Read the model definition and answer for the solid it produces. Units are mm, in the model's axes. A direction names the side the tool comes from. Give positions to 0.01 mm unless a question says otherwise; leave off trailing zeros. Order: outer loops, then holes, each group sorted by start corner. A loop starts at its lowest first (then second) coordinate and runs counter-clockwise, first axis right, second up. Notation, with made-up numbers: (57.25, 76.5) - (86.25, 76.5) arc R23 cw to (86.25, 87.5) - close; hole circle Ø4 at (6.5, 35.25). An arc over 180 degrees is marked (long way). Return JSON: item names as keys, results as strings.
```python
from build123d import *

# Parameters (mm, degrees)
SKETCH_1_W          = 45
SKETCH_1_H          = 80
EXTRUDE_1_DEPTH     = 6
CUT_EXTRUDE_2_DEPTH = 84.320165626
FILLET_10_R         = 2
M3X0_52_D           = 2.5
M3X0_52_DEPTH       = 8.5
M3X0_52_TIP         = 0.751075774
M3X0_51_D           = 2.5
M3X0_51_DEPTH       = 8.5
M3X0_51_TIP         = 0.751075774


with BuildPart() as part:
    # Эскиз1 → Бобышка-Вытянуть1 (new body)
    with BuildSketch(Plane(origin=(0, 0, 0), x_dir=(1, 0, 0), z_dir=(0, 1, 0))):
        with Locations((0, -40)):
            Rectangle(SKETCH_1_W, SKETCH_1_H)
    extrude(amount=EXTRUDE_1_DEPTH)

    # Эскиз13 → Вырез-Вытянуть2 (cut, through all)
    with BuildSketch(Plane(origin=(0, 6, 0), x_dir=(1, 0, 0), z_dir=(0, 1, 0))):
        Polygon((-18.5, -8), (18.5, -8), (-18.5, -38), align=None)
        Polygon((18.5, -72), (-18.5, -42), (-18.5, -72), align=None)
        Polygon((18.5, -13.149623941), (-14.615463806, -40), (18.5, -66.850376059), align=None)
    extrude(amount=-CUT_EXTRUDE_2_DEPTH, mode=Mode.SUBTRACT)

    # Скругление10
    fillet_10_edges = [part.edges().sort_by_distance(p)[0] for p in [
        (18.5, 3, 72),
        (-18.5, 3, 72),
        (-18.5, 3, 42),
        (-18.5, 3, 38),
        (-18.5, 3, 8),
        (18.5, 3, 8),
        (18.5, 3, 13.149623941),
        (18.5, 3, 66.850376059),
        (-14.615463806, 3, 40),
    ]]
    fillet(fillet_10_edges, radius=FILLET_10_R)

    # Отверстие обработанное метчиком M3x0.52
    with Locations(Plane(origin=(0, 0, 0), x_dir=(-1, 0, 0), z_dir=(0, 0, -1))):
        with Locations((-13.5, 3), (-4.5, 3), (4.5, 3), (13.5, 3)):
            Hole(M3X0_52_D / 2, depth=M3X0_52_DEPTH)
            with Locations((0, 0, -(M3X0_52_DEPTH + M3X0_52_TIP / 2))):  # 118° drill point
                Cone(0, M3X0_52_D / 2, M3X0_52_TIP, mode=Mode.SUBTRACT)

    # Отверстие обработанное метчиком M3x0.51
    with Locations(Plane.XY.offset(80)):
        with Locations((-13.5, 3), (-4.5, 3), (4.5, 3), (13.5, 3)):
            Hole(M3X0_51_D / 2, depth=M3X0_51_DEPTH)
            with Locations((0, 0, -(M3X0_51_DEPTH + M3X0_51_TIP / 2))):  # 118° drill point
                Cone(0, M3X0_51_D / 2, M3X0_51_TIP, mode=Mode.SUBTRACT)


solid = part.part
```
Q1. Consider L1, parallel to Z at x = -16.5, y = 1.5; L2, parallel to Z at x = 11.5, y = 2; L3, parallel to Y at x = 4.5, z = 4. Determine where each line is inside the solid, lowest interval first.
Values:
{"L1": "z = 0 to 8, 35.8 to 44.2, 72 to 80", "L2": "z = 0 to 8, 13.68 to 18.83, 61.17 to 66.32, 72 to 80", "L3": "y = 0 to 1.75, 4.25 to 6"}
Q2. A cutting plane is placed at B-B (x = -4.5). Write down the section's boundary in (y, z), and give its area (3 significant figures).
Values:
{"outline": "(0, 0) - (1.75, 0) - (1.75, 8) - (0, 8) - close; (0, 26.65) - (6, 26.65) - (6, 31.8) - (0, 31.8) - close; (0, 48.2) - (6, 48.2) - (6, 53.35) - (0, 53.35) - close; (0, 72) - (1.75, 72) - (1.75, 80) - (0, 80) - close; (4.25, 0) - (6, 0) - (6, 8) - (4.25, 8) - close; (4.25, 72) - (6, 72) - (6, 80) - (4.25, 80) - close", "area": "118 mm²"}
Q3. Given pin 1 (3 mm diameter, centred on x = 13.5, y = 3, fed in from -Z); pin 2 (2 mm diameter, centred on x = 13.5, y = 3, fed in from +Z); pin 3 (2 mm diameter, centred on x = -13.5, y = 3, fed in from -Z), each flat-ended and moving along its own axis, determine where each tip first touches the part or whether it passes through.
Values:
{"pin 1": "stops at z = 0", "pin 2": "stops at z = 71.35", "pin 3": "stops at z = 33.14"}
Q4. Determine the mould class of faces 6 (the flat face through (-2, 3, 8)), 7 (the flat face through (22.5, 3, 41)), 8 (the flat face through (0, 3, 0)) for opening direction Z: released by +Z, released by -Z, zero draft, split by the parting line, or undercut.
Values:
{"face 6": "undercut", "face 7": "zero draft", "face 8": "released by -Z"}
Q5. A cutting plane is placed at D-D (x = -9). Write down the section's boundary in (y, z).
Values:
{"outline": "(0, 0) - (6, 0) - (6, 8) - (0, 8) - close; (0, 30.3) - (6, 30.3) - (6, 35.45) - (0, 35.45) - close; (0, 44.55) - (6, 44.55) - (6, 49.7) - (0, 49.7) - close; (0, 72) - (6, 72) - (6, 80) - (0, 80) - close"}
Q6. A cutting plane is placed at A-A (y = 5.25). Write down the section's boundary in (x, z), and give its area (3 significant figures).
Values:
{"outline": "(-22.5, 0) - (22.5, 0) - (22.5, 80) - (-22.5, 80) - close; hole (-18.5, 10) arc R2 ccw to (-16.5, 8) - (12.86, 8) arc R2 ccw to (14.12, 11.55) - (-15.24, 35.36) arc R2 ccw to (-18.5, 33.8) - close; hole (-18.5, 46.2) arc R2 ccw to (-15.24, 44.64) - (14.12, 68.45) arc R2 ccw to (12.86, 72) - (-16.5, 72) arc R2 ccw to (-18.5, 70) - close; hole (-12.7, 38.45) - (15.24, 15.79) arc R2 ccw to (18.5, 17.35) - (18.5, 62.65) arc R2 ccw to (15.24, 64.21) - (-12.7, 41.55) arc R2 ccw to start", "area": "1,630 mm²"}
Q7. For faces 1 (the flat face through (-5, 6, 48)), 2 (the cylindrical face through (-5.421, 3.845, 4.056)), 3 (the cylindrical face through (5.421, 3.845, 75.944)), 4 (the flat face through (-18.5, 3, 58)), 5 (the flat face through (-5, 0, 48)), determine the directions among +Z, -Z, +X, -X, +Y, -Y from which every point of the face is accessible in a straight line to the end or side of a thin tool.
Values:
{"face 1": "+Z, -Z, +X, -X, +Y", "face 2": "-Z", "face 3": "+Z", "face 4": "+Y, -Y", "face 5": "+Z, -Z, +X, -X, -Y"}
Q8. A cutting plane is placed at C-C (z = 6.5). Write down the section's boundary in (x, y), and give its area (3 significant figures).
Values:
{"outline": "(-22.5, 0) - (22.5, 0) - (22.5, 6) - (-22.5, 6) - close; hole circle Ø2.5 at (-13.5, 3); hole circle Ø2.5 at (-4.5, 3); hole circle Ø2.5 at (4.5, 3); hole circle Ø2.5 at (13.5, 3)", "area": "250 mm²"}
